The listing builds one solid part. Answer for the finished solid, in the listing's coordinates (mm). Face numbers are marked on the shaded views. A direction names the side the tool comes from. Coordinates: 2 decimals unless noted, no trailing zeros. Write each loop counter-clockwise with the first axis right and the second up, starting at its lowest first coordinate (ties: lowest second). Pieces come first, ordered by that corner, then holes. Notation, with made-up numbers: M 3.5,-37 L 49.5,-37 A22 cw 49.5,-8 Z; hole C -37,56 d5. An arc over 180 degrees is marked long. Answer as CSV lines item,"result".
Autodesk Inventor part; units mm, degrees
ref_plane "YZ Plane" through (0, 0, 0) normal (1, 0, 0) x (0, 1, 0)
ref_plane "XZ Plane" through (0, 0, 0) normal (0, 1, 0) x (-1, 0, 0)
ref_plane "XY Plane" through (0, 0, 0) normal (0, 0, 1) x (1, 0, 0)
sketch "スケッチ1" plane through (0, 0, 0) normal (0, 1, 0) x (-1, 0, 0)
  line L0 (135, 77.9423) -> (-135, 77.9423)
  line L1 (-135, 77.9423) -> (0, -155.8846)
  line L2 (0, -155.8846) -> (135, 77.9423)
  line L3 (135, 77.9423) -> (-67.5, -38.9711) construction
  line L4 (75, 77.9423) -> (105, 25.9808)
  line L5 (-105, 25.9808) -> (-75, 77.9423)
  line L6 (30, -103.923) -> (-30, -103.923)
  line L7 (77.8868, 82.9423) -> (0, 82.9423)
  line L8 (77.8868, 82.9423) -> (94.3301, 54.4615)
  line L9 (0, 0) -> (0, 82.9423) construction
  line L10 (-77.8868, 82.9423) -> (0, 82.9423)
  line L11 (-77.8868, 82.9423) -> (-94.3301, 54.4615)
  line L12 (-110.7735, 25.9808) -> (-94.3301, 54.4615)
  line L13 (-110.7735, 25.9808) -> (-71.8301, -41.4711)
  line L14 (-32.8868, -108.923) -> (-71.8301, -41.4711)
  line L15 (-32.8868, -108.923) -> (0, -108.923)
  line L16 (32.8868, -108.923) -> (0, -108.923)
  line L17 (32.8868, -108.923) -> (71.8301, -41.4711)
  line L18 (110.7735, 25.9808) -> (71.8301, -41.4711)
  line L19 (110.7735, 25.9808) -> (94.3301, 54.4615)
  line L20 (30, -108.923) -> (30, -103.923)
  line L21 (-30, -108.923) -> (-30, -103.923)
  line L22 (-30, -103.923) -> (30, -103.923)
  dimension "d0" = 270
  dimension "d1" = 60
  dimension "d4" = 360
  dimension "d6" = 5
  dimension "d7" = 5
  dimension "d10" = 360
extrude "押し出し2" add sketch "スケッチ1" along normal blind 20 contours L4 L2 L6 L1 L5 L0
sketch "スケッチ2" plane through (0, 20, 0) normal (0, 1, 0) x (1, 0, 0)
  line L0 (-75, -77.9423) -> (75, -77.9423)
  line L1 (-29, -77.9423) -> (29, -77.9423)
  line L2 (29, -77.9423) -> (29, -51.9423)
  line L3 (29, -51.9423) -> (-29, -51.9423)
  line L4 (-29, -51.9423) -> (-29, -77.9423)
  point P0 (0, 0)
  point P1 (0, -51.9423)
  point P2 (0, -77.9423)
  dimension "d16" = 26
  dimension "d17" = 58
extrude "押し出し3" cut sketch "スケッチ2" against normal blind 20
pattern_circular "円形状パターン1" count 3 over 360 about axis through (0, -10, 0) along (0, 1, 0) of "押し出し3"
properties part number "base_flame"
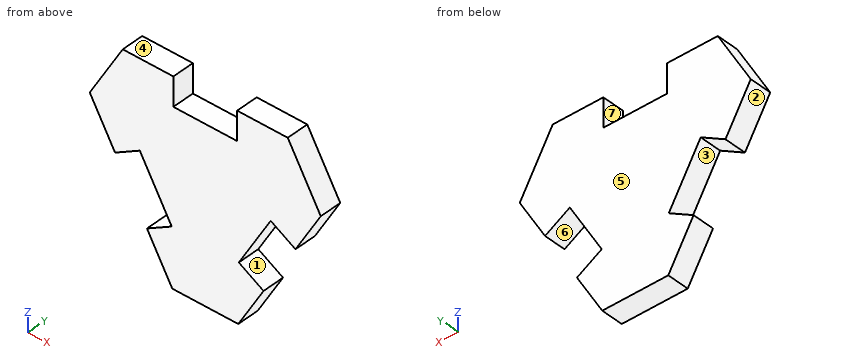
Q1. Find section D-D (z = -86.5). Give the vertices of the cut face in (x, y).
Output:
outline,"M -40.06,0 L 40.06,0 L 40.06,20 L -40.06,20 Z"
Q2. Flat-ended cylindrical pins translate along their axes: pin 1 Ø2 at (x, y) = (-50, 16.5) entering from -Z; pin 2 Ø1 at (y, z) = (8, -53.5) entering from -X; pin 3 Ø12 at (y, z) = (3.5, -49.5) entering from -X. Find the tip coordinate at first contact, or state that the pin passes through.
Output:
pin 1,"z = -71.01"
pin 2,"x = -35.53"
pin 3,"x = -38.13"
Q3. The mould has two halves that part along Z. Classify the marked faces 1, 2, 3 and 4: pulls with the +Z half, pulls with the -Z half, needs draft (parallel to the pull), parting line crosses it, or undercut.
Output:
face 1,"undercut"
face 2,"pulls with the -Z half"
face 3,"undercut"
face 4,"pulls with the +Z half"
Q4. For the marked faces 5, 6 and 7, determine the directions among +Z, -Z, +X, -X, +Y, -Y from which every point of the face is accessible in a straight line to the end or side of a thin tool.
Output:
face 5,"+Z, -Z, +X, -X, +Y"
face 6,"-Z, +Y, -Y"
face 7,"+Z, +Y, -Y"
Q5. Straight lines are drawn through the part: line 1 (X direction, y = 11, z = -9); line 2 (Z direction, x = 12, y = 3.5); line 3 (X direction, y = 9.5, z = -12). For each, find the intervals that lie inside material, in ascending order.
Output:
line 1,"-84.8 to -73.59, -54.78 to 54.78, 73.59 to 84.8"
line 2,"-103.92 to 51.94"
line 3,"-83.07 to -78.78, -53.05 to 53.05, 78.78 to 83.07"
Q6. Find section C-C (y = 15). Give the vertices of the cut face in (x, z).
Output:
outline,"M -105,25.98 L -82,-13.86 L -59.48,-0.86 L -30.48,-51.09 L -53,-64.09 L -30,-103.92 L 30,-103.92 L 53,-64.09 L 30.48,-51.09 L 59.48,-0.86 L 82,-13.86 L 105,25.98 L 75,77.94 L 29,77.94 L 29,51.94 L -29,51.94 L -29,77.94 L -75,77.94 Z"
Q7. Find section A-A (x = -34). Give the vertices of the cut face in (y, z).
Output:
outline,"M 0,-96.99 L 20,-96.99 L 20,-53.12 L 0,-53.12 Z; M 0,-44.99 L 20,-44.99 L 20,77.94 L 0,77.94 Z"
Q8. Find section B-B (z = -8.5). Give the vertices of the cut face in (x, y), and give its area (3 significant figures).
Output:
outline,"M -85.09,0 L -72.72,0 L -72.72,20 L -85.09,20 Z; M -55.07,0 L 55.07,0 L 55.07,20 L -55.07,20 Z; M 72.72,0 L 85.09,0 L 85.09,20 L 72.72,20 Z"
area,"2,700 mm2"
